Geometry: final body of the model. Coordinates: model frame, mm. Give positions to 0.01 mm unless a question says otherwise; leave off trailing zeros. Write each loop counter-clockwise with the first axis right and the second up, starting at its lowest first coordinate (ties: lowest second). Pieces come first, ordered by that corner, then holes.
Autodesk Inventor part; units mm, degrees
ref_plane "YZ Plane" through (0, 0, 0) normal (1, 0, 0) x (0, 1, 0)
ref_plane "XZ Plane" through (0, 0, 0) normal (0, 1, 0) x (-1, 0, 0)
ref_plane "XY Plane" through (0, 0, 0) normal (0, 0, 1) x (1, 0, 0)
sketch "Sketch1" plane through (0, 0, 0) normal (0, 1, 0) x (-1, 0, 0)
  line L0 (46.3062, 23.9021) -> (20.9062, 23.9021)
  line L1 (20.9062, 23.9021) -> (20.9062, -26.8979)
  line L2 (15.3051, -52.2979) -> (46.3062, -52.2979)
  line L3 (46.3062, -52.2979) -> (46.3062, 23.9021)
  line L4 (46.3062, -52.2979) -> (-29.8938, -52.2979)
  line L5 (-29.8938, -52.2979) -> (-29.8938, -26.8979)
  line L6 (-29.8938, -26.8979) -> (20.9062, -26.8979)
  line L7 (46.3062, -26.8979) -> (46.3062, -52.2979)
  point P0 (0, 0)
  dimension "d0" = 25.4
  dimension "d1" = 25.4
  dimension "d2" = 76.2
  dimension "d3" = 76.2
extrude "Extrusion1" add sketch "Sketch1" along normal blind 1.5875
sketch "Sketch2" plane through (0, 1.5875, 0) normal (0, 1, 0) x (1, 0, 0)
  line L0 (-46.3062, -23.9021) -> (-20.9062, -23.9021)
  line L1 (-46.3062, 52.2979) -> (-46.3062, -23.9021)
  line L2 (-20.9062, -23.9021) -> (-20.9062, 26.8979)
  point P0 (0, 0)
  point P1 (-39.9562, -17.5521)
  point P2 (-27.2562, -4.8521)
  point P3 (-39.9562, 7.8479)
  point P4 (-27.2562, 20.5479)
  dimension "d6" = 6.35
  dimension "d7" = 6.35
  dimension "d8" = 6.35
  dimension "d9" = 12.7
  dimension "d10" = 12.7
  dimension "d11" = 6.35
  dimension "d12" = 12.7
  dimension "d13" = 6.35
hole "Hole1" at (-39.9562, 1.5875, 17.5521) at (-27.2562, 1.5875, 4.8521) at (-39.9562, 1.5875, -7.8479) at (-27.2562, 1.5875, -20.5479) direction (0, -1, 0) diameter 4.7625 depth 25.4 tip angle 118
sketch "Sketch3" plane through (0, 1.5875, 0) normal (0, 1, 0) x (1, 0, 0)
  line L0 (29.8938, 26.8979) -> (29.8938, 52.2979)
  line L1 (-20.9062, 26.8979) -> (29.8938, 26.8979)
  line L2 (29.8938, 52.2979) -> (-46.3062, 52.2979)
  point P0 (0, 0)
  point P1 (-14.5562, 45.9479)
  point P2 (-1.8562, 33.2479)
  point P3 (23.5438, 33.2479)
  point P4 (10.8438, 45.9479)
  dimension "d21" = 6.35
  dimension "d22" = 6.35
  dimension "d23" = 12.7
  dimension "d24" = 6.35
  dimension "d25" = 12.7
  dimension "d26" = 6.35
  dimension "d27" = 12.7
  dimension "d28" = 6.35
hole "Hole2" at (-14.5562, 1.5875, -45.9479) at (-1.8562, 1.5875, -33.2479) at (23.5438, 1.5875, -33.2479) at (10.8438, 1.5875, -45.9479) direction (0, -1, 0) diameter 4.7625 depth 25.4 tip angle 118
equation "\"d0\" = ElvBeamWidth"
equation "\"d1\" = ElvBeamWidth"
equation "\"d2\" = ElvRivetPlateLength"
equation "\"d3\" = ElvRivetPlateLength"
equation "\"d4\" = ElvWallWidth"
equation "\"ElvCrossBeamLength\" = 304.8"
equation "\"ElvFixedBeamLength\" = 990.6"
equation "\"ElvMiddleBeamLength\" = 990.6"
equation "\"ElvFrontBeamLength\" = 990.6"
equation "\"ElvEndEffectLength\" = 431.8"
equation "\"ElvBeamWidth\" = 25.4"
equation "\"ElvWallWidth\" = 1.5875"
equation "\"ElvDelWidth\" = 18.542"
equation "\"ElvDelHeight\" = 101.6"
equation "\"ElvDelFrontTabLength\" = 6.35"
equation "\"ElvDelDepth\" = 6.35"
equation "\"ElvTopBeamLength\" = 457.2"
equation "\"ElvHoleFromFront\" = 25.4"
equation "\"ElvHoleFromMid\" = 38.1"
equation "\"ElvHoleFromFixed\" = 50.8"
equation "\"ElvHoleFromBottom\" = 38.1"
equation "\"ElvRivetPlateLength\" = 76.2"
equation "\"ElvDelMiddleTabLength\" = 6.35"
properties part number "elvRivetPlate"
Q1. Pin query (flat end, axial travel): P1, Ø0.5, axis at y = 1, z = -7.5, coming from the +X side; P2, Ø4.5, axis at x = -14.56, z = -45.95, coming from the +Y side. Return the tip coordinate at first contact, or that it passes through.
Filled sheet:
P1: stops at x = -20.91
P2: passes through
Q2. Section A-A on z = -9. Output: boundary loops of the cut face in (x, y).
Filled sheet:
outline: (-46.31, 0) - (-42.04, 0) - (-42.04, 1.59) - (-46.31, 1.59) - close; (-37.87, 0) - (-20.91, 0) - (-20.91, 1.59) - (-37.87, 1.59) - close
Q3. Pull-direction query (X, two-part tool) for faces 1 (the cylindrical face through (-37.63, 0.78, 17.04)), 2 (the flat face through (-25, 0, -22)); classes: released by +X, released by -X, zero draft, split by the parting line, or undercut.
Filled sheet:
face 1: undercut
face 2: zero draft
Q4. Ray query, line 1 along Z through (x, y) = (-27.5, 0.7); line 2 along X through (y, z) = (1.25, -8); line 3 along X through (y, z) = (1.2, -35). Return the intervals inside material, ascending.
Filled sheet:
line 1: z = -52.3 to -22.92, -18.18 to 2.48, 7.22 to 23.9
line 2: x = -46.31 to -42.33, -37.58 to -20.91
line 3: x = -46.31 to -3.47, -0.24 to 21.93, 25.16 to 29.89
Q5. Section B-B on y = 0.6. Count the separate pieces of the cut face and the enclosed holes in it, plus the area to 3 significant figures.
Filled sheet:
separate pieces: 1
enclosed holes: 8
area: 3,080 mm2
Q6. Section D-D on z = 9.5. Output: boundary loops of the cut face in (x, y), plus the area to 3 significant figures.
Filled sheet:
outline: (-46.31, 0) - (-20.91, 0) - (-20.91, 1.59) - (-46.31, 1.59) - close
area: 40.3 mm2
Q7. Section C-C on x = 3. Output: boundary loops of the cut face in (y, z).
Filled sheet:
outline: (0, -52.3) - (1.59, -52.3) - (1.59, -26.9) - (0, -26.9) - close
